from build123d import *

# Parameters (mm, degrees)
SKETCH_1_W               = 3.2
SKETCH_1_H               = 3.2
SKETCH_1_W_2             = 1.76
SKETCH_1_H_2             = 1.76
EXTRUDE_1_DEPTH          = 7
SKETCH_2_W               = 3.2
SKETCH_2_H               = 3.2
EXTRUDE_2_DEPTH          = 1.2
EXTRUDE_3_DEPTH          = 2.6
CUT_EXTRUDE_1_DEPTH      = 1.2
SKETCH_5_W               = 5.2
SKETCH_5_H               = 3.2
EXTRUDE_4_DEPTH          = 1.2
CUT_EXTRUDE_2_DEPTH      = 9.124038405
CUT_EXTRUDE_2_DEPTH_BACK = 9.124038405
SKETCH_6_R               = 0.35


with BuildPart() as part:
    # 草图1 → 凸台-拉伸1 (new body)
    with BuildSketch(Plane(origin=(0, 0, 0), x_dir=(0, 0, -1), z_dir=(1, 0, 0))):
        Rectangle(SKETCH_1_W, SKETCH_1_H)
        Rectangle(SKETCH_1_W_2, SKETCH_1_H_2, mode=Mode.SUBTRACT)
    extrude(amount=EXTRUDE_1_DEPTH)

    # 草图2 → 凸台-拉伸2 (add)
    with BuildSketch(Plane.ZY):
        Rectangle(SKETCH_2_W, SKETCH_2_H)
    extrude(amount=EXTRUDE_2_DEPTH)

    # 草图3 → 凸台-拉伸3 (add, symmetric)
    with BuildSketch(Plane.XY):
        with BuildLine():
            Line((-1.2, -1.1), (-1.2, 1.1))
            Line((-1.2, 1.1), (-2.52, 1.1))
            ThreePointArc((-2.52, 1.1), (-2.165084685, 0.600122548), (-2.039803903, 0))
            ThreePointArc((-2.039803903, 0), (-2.165084685, -0.600122548), (-2.52, -1.1))
            Line((-2.52, -1.1), (-1.2, -1.1))
        make_face()
        with BuildLine():
            ThreePointArc((-2.039803903, 0), (-2.165084685, 0.600122548), (-2.52, 1.1))
            Line((-2.52, 1.1), (-2.52, -1.1))
            ThreePointArc((-2.52, -1.1), (-2.165084685, -0.600122548), (-2.039803903, 0))
        make_face()
        with BuildLine():
            Line((-2.52, -1.1), (-2.52, 1.1))
            ThreePointArc((-2.52, 1.1), (-5.039803903, 0), (-2.52, -1.1))
        make_face()
        with BuildLine():
            ThreePointArc((-2.039803903, 0), (-2.165084685, 0.600122548), (-2.52, 1.1))
            Line((-2.52, 1.1), (-2.52, -1.1))
            ThreePointArc((-2.52, -1.1), (-2.165084685, -0.600122548), (-2.039803903, 0))
        make_face()
        with BuildLine():
            Line((-2.52, -1.1), (-2.52, 1.1))
            ThreePointArc((-2.52, 1.1), (-5.039803903, 0), (-2.52, -1.1))
        make_face()
    extrude(amount=EXTRUDE_3_DEPTH, both=True)

    # 草图4 → 切除-拉伸1 (cut, symmetric)
    with BuildSketch(Plane.XY):
        with BuildLine():
            Line((-1.2, 1.1), (-2.52, 1.1))
            ThreePointArc((-2.52, 1.1), (-5.039803903, 0), (-2.52, -1.1))
            Line((-2.52, -1.1), (-1.2, -1.1))
            Line((-1.2, -1.1), (-1.2, 1.1))
        make_face()
    extrude(amount=CUT_EXTRUDE_1_DEPTH, both=True, mode=Mode.SUBTRACT)

    # 草图5 → 凸台-拉伸4 (add)
    with BuildSketch(Plane(origin=(-1.2, 0, 0), x_dir=(0, 0, -1), z_dir=(1, 0, 0))):
        Rectangle(SKETCH_5_W, SKETCH_5_H)
    extrude(amount=EXTRUDE_4_DEPTH)

    # 草图6 → 切除-拉伸2 (cut, two sides: drawn at the far end of the back side and taken through both)
    with BuildSketch(Plane(origin=(0, 0, 1.2), x_dir=(-1, 0, 0), z_dir=(0, 0, -1)).offset(-CUT_EXTRUDE_2_DEPTH_BACK)):
        with Locations((3.539803903, 0)):
            Circle(SKETCH_6_R)
    extrude(amount=CUT_EXTRUDE_2_DEPTH + CUT_EXTRUDE_2_DEPTH_BACK, mode=Mode.SUBTRACT)


solid = part.part
Model file for the job. Use its own axes, mm. A direction names the side the tool comes from. Round coordinates to 2 decimals unless told otherwise and drop trailing zeros. Order: outer loops, then holes, each group sorted by start corner. A loop starts at its lowest first (then second) coordinate and runs counter-clockwise, first axis right, second up.
(1) Band-saw the part on B-B (y = -1.3). List the corners of the cut face in (x, z).
(2) Band-saw the part on D-D (z = -1). List the corners of the cut face in (x, y), then the cut area to 3 significant figures.
(3) Drill centre lines: line 1 (X direction, y = 0, z = 1.55); line 2 (Z direction, x = 1.5, y = -0.55); line 3 (Z direction, x = -3.5, y = -0.75). Where is each one in solid material? Low to high.
(4) Band-saw the part on C-C (z = -0.25). List the corners of the cut face in (x, y), then the cut area to 3 significant figures.
(5) Band-saw the part on A-A (x = 4). List the corners of the cut face in (y, z).
(6) 3-axis set-ups, long thin cutter, end or side, ignore diameter. For faces 1 (the face through (-3, 0, -1.2)), 2 (the face through (3, 0.88, 0)), 3 (the face through (0, 0, -2)), 4 (the face through (-2, 1.1, 2)), 5 (the face through (0, 0, 2)): which of +Z, -Z, +X, -X, +Y, -Y reach the whole face in a straight line?
(7) Pull direction Z, two halves, no side cores. Call faces 6 (the face through (0, 0, 0)), 7 (the face through (3, -1.6, 0)), 8 (the face through (-3, 0, -2.6)): released by +Z, released by -Z, zero draft, split by the parting line, or undercut.
(8) Pin check, flat tips, straight feed: pin 1 (0.9 mm diameter, centred on x = 3, y = -0.5, fed in from -Z); pin 2 (1.5 mm diameter, centred on x = -2, z = -2, fed in from -Y); pin 3 (2 mm diameter, centred on x = -3, z = -0.5, fed in from -Y). Stop position of each tip, or through.
Verdict:
1. outline: (-4.29, -2.6) - (-2.79, -2.6) - (-2.79, -1.2) - (-4.29, -1.2) - close; (-4.29, 1.2) - (-2.79, 1.2) - (-2.79, 2.6) - (-4.29, 2.6) - close; (-1.2, -2.6) - (0, -2.6) - (0, -1.6) - (7, -1.6) - (7, 1.6) - (0, 1.6) - (0, 2.6) - (-1.2, 2.6) - close
2. outline: (-1.2, -1.6) - (7, -1.6) - (7, 1.6) - (-1.2, 1.6) - close
2. area: 26.2 mm2
3. line 1: x = -5.04 to -3.89, -3.19 to 7
3. line 2: z = -1.6 to -0.88, 0.88 to 1.6
3. line 3: z = -2.6 to -1.2, 1.2 to 2.6
4. outline: (-1.2, -1.6) - (7, -1.6) - (7, -0.88) - (0, -0.88) - (0, 0.88) - (7, 0.88) - (7, 1.6) - (-1.2, 1.6) - close
4. area: 13.9 mm2
5. outline: (-1.6, -1.6) - (1.6, -1.6) - (1.6, 1.6) - (-1.6, 1.6) - close; hole (-0.88, -0.88) - (0.88, -0.88) - (0.88, 0.88) - (-0.88, 0.88) - close
6. face 1: -X, +Y, -Y
6. face 2: +X
6. face 3: -Z, +X, +Y, -Y
6. face 4: +Z, -Z, +Y
6. face 5: +Z, +X, +Y, -Y
7. face 6: undercut
7. face 7: zero draft
7. face 8: released by -Z
8. pin 1: stops at z = -1.6
8. pin 2: stops at y = -1.28
8. pin 3: stops at y = -1.5
